Input: dimensioned drawing with shaded views. Units: mm. Origin: part minimum x, y, z. A direction names the side the tool comes from. Round coordinates to 2 decimals unless told otherwise and drop trailing zeros. Loops run counter-clockwise (first coordinate to the right, second up) from the corner with the lowest first, then second, coordinate; pieces in that order, holes last. Notation, with made-up numbers: (84, 61) - (133, 61) arc R15 ccw to (133, 77) - close; hole circle Ø5 at (66, 44). An arc over 180 degrees is marked (long way). Answer as CSV lines item,"result".
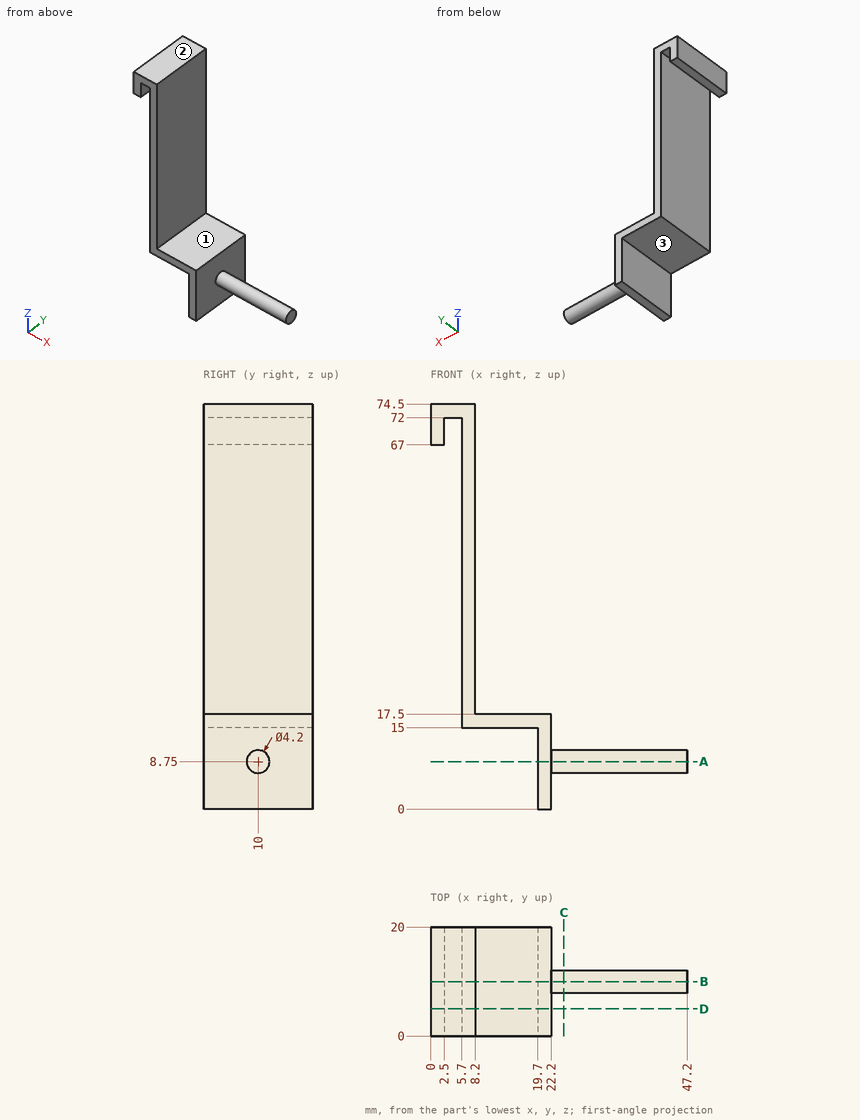
(1) Section D-D (y = 5). Output: boundary loops of the cut face in (x, z).
Findings below:
outline,"(0, 67) - (2.5, 67) - (2.5, 72) - (5.7, 72) - (5.7, 15) - (19.7, 15) - (19.7, 0) - (22.2, 0) - (22.2, 17.5) - (8.2, 17.5) - (8.2, 74.5) - (0, 74.5) - close"
(2) Pin query (flat end, axial travel): P1, Ø12, axis at x = 37, y = 13, coming from the +Z side; P2, Ø4, axis at x = 11.5, y = 10.5, coming from the -Z side; P3, Ø4, axis at y = 4, z = 50, coming from the -X side. Return the tip coordinate at first contact, or that it passes through.
Findings below:
P1,"z = 10.85"
P2,"z = 15"
P3,"x = 5.7"
(3) Section C-C (x = 24.5). Output: boundary loops of the cut face in (y, z), and give its area (3 significant figures).
Findings below:
outline,"circle Ø4.2 at (10, 8.75)"
area,"13.9 mm2"
(4) Section B-B (y = 10). Output: boundary loops of the cut face in (x, z).
Findings below:
outline,"(0, 67) - (2.5, 67) - (2.5, 72) - (5.7, 72) - (5.7, 15) - (19.7, 15) - (19.7, 0) - (22.2, 0) - (22.2, 6.65) - (47.2, 6.65) - (47.2, 10.85) - (22.2, 10.85) - (22.2, 17.5) - (8.2, 17.5) - (8.2, 74.5) - (0, 74.5) - close"
(5) Material intervals for line 1 along X through (y, z) = (7, 25); line 2 along Z through (x, y) = (11, 9.75); line 3 along Z through (x, y) = (2, 17.75), sorted ascending.
Findings below:
line 1,"5.7 to 8.2"
line 2,"15 to 17.5"
line 3,"67 to 74.5"
(6) Access query for the marked faces 1, 2 and 3. Directions: +Z, -Z, +X, -X, +Y, -Y. A direction counts if a zero-diameter tool reaches every point of the face in a straight line with its end or side. Return the directions, or none.
Findings below:
face 1,"+Z, +X, +Y, -Y"
face 2,"+Z, +X, -X, +Y, -Y"
face 3,"-Z, -X, +Y, -Y"
(7) Section A-A (z = 8.75). Output: boundary loops of the cut face in (x, y), and give its area (3 significant figures).
Findings below:
outline,"(19.7, 0) - (22.2, 0) - (22.2, 7.9) - (47.2, 7.9) - (47.2, 12.1) - (22.2, 12.1) - (22.2, 20) - (19.7, 20) - close"
area,"155 mm2"
